```python
from build123d import *

# Parameters (mm, degrees)
F1_DEPTH = 63.5
F0_W     = 25.4
F0_H     = 19.05
F2_DEPTH = 25.4
F3_DEPTH = 7.9375
F4_R     = 6.35


with BuildPart() as f1:
    # F0 (on Top) → F1 (new body, symmetric)
    with BuildSketch(Plane.XY):
        Polygon((-41.275, -9.525), (41.275, -9.525), (41.275, 9.525), (22.225, 9.525), (-41.275, 9.525), align=None)
    extrude(amount=F1_DEPTH, both=True)

    # F0 (on Top) → F2 (join, symmetric)
    with BuildSketch(Plane.XY):
        with BuildLine():
            Line((22.225, 9.525), (41.275, 9.525))
            Line((41.275, 9.525), (41.275, 42.8379135305))
            ThreePointArc((41.275, 42.8379135305), (41.8183842247, 42.8658756442), (42.3624075254, 42.8752))
            Line((42.3624075254, 42.8752), (60.325, 42.8752))
            Line((60.325, 42.8752), (60.325, 61.9252))
            Line((60.325, 61.9252), (42.3624075254, 61.9252))
            add(Edge.make_bspline(
                [(41.3653767795, 61.9109655988), (41.6979264338, 61.916873269), (42.0302788073, 61.9216177836), (42.3624075254, 61.9252)],
                knots=[97.8694671613, 97.8694671613, 97.8694671613, 97.8694671613, 98.6964887806, 98.6964887806, 98.6964887806, 98.6964887806], degree=3))
            ThreePointArc((41.3653767795, 61.9109655988), (31.324788218, 60.1351752531), (22.225, 55.5350986883))
            Line((22.225, 55.5350986883), (22.225, 9.525))
        make_face()
        with Locations((73.025, 52.4002)):
            Rectangle(F0_W, F0_H)
    extrude(amount=F2_DEPTH, both=True)

    # F0 (on Top) → F3 (join, symmetric)
    with BuildSketch(Plane.XY):
        with BuildLine():
            add(Edge.make_bspline(
                [(-41.275, 9.525), (-40.1050332587, 44.223586325), (2.0115597622, 61.211853837), (41.3653767795, 61.9109655988)],
                knots=[0, 0, 0, 0, 97.8694671613, 97.8694671613, 97.8694671613, 97.8694671613], degree=3))
            Line((-41.275, 9.525), (22.225, 9.525))
            Line((22.225, 9.525), (22.225, 55.5350986883))
            ThreePointArc((22.225, 55.5350986883), (31.324788218, 60.1351752531), (41.3653767795, 61.9109655988))
        make_face()
    extrude(amount=F3_DEPTH, both=True)

    # F4
    f4_edges = [f1.edges().sort_by_distance(p)[0] for p in [
        (41.275, 0, 63.5),
        (-41.275, 0, 63.5),
        (-41.275, 0, -63.5),
        (41.275, 0, -63.5),
    ]]
    fillet(f4_edges, radius=F4_R)

    # F0 (on Top) → F5 (revolve)
    with BuildSketch(Plane.XY):
        Polygon((85.725, 61.9252), (85.725, 42.8752), (85.725, 38.1), (111.125, 38.1), (111.125, 66.675), (85.725, 66.675), align=None)
    revolve(axis=Axis((85.725, 52.3875, 0), (0, 1, 0)))


solid = f1.part
```
Verification items for the finished model (mm, model axes). A direction names the side the tool comes from. Coordinates: 2 decimals unless noted, no trailing zeros. Write each loop counter-clockwise with the first axis right and the second up, starting at its lowest first coordinate (ties: lowest second). Pieces come first, ordered by that corner, then holes. Notation, with made-up numbers: (2, -7.5) - (57, -7.5) arc R27 ccw to (57, 19.5) - close; hole circle Ø11 at (18, -15.5). An arc over 180 degrees is marked (long way). Write item = value, one per line.
Q1. Cross-section at C-C (x = 68.5). Enter the section's corners in (y, z) (3 decimals), plus the area to 3 significant figures.
Answer:
outline = (38.1, -18.667) - (42.875, -18.667) - (42.875, -25.4) - (61.925, -25.4) - (61.925, -18.667) - (66.675, -18.667) - (66.675, 18.667) - (61.925, 18.667) - (61.925, 25.4) - (42.875, 25.4) - (42.875, 18.667) - (38.1, 18.667) - close
area = 1,320 mm²
Q2. Material ranges on L1, parallel to Y at x = -23.5, z = -13 (3 decimals); L2, parallel to Z at x = 40, y = 42.5; L3, parallel to Z at x = -14, y = 18, recorded low to high. Write a range as from..to.
Answer:
L1 = -9.525..9.525
L2 = -25.4..25.4
L3 = -7.94..7.94
Q3. Cross-section at A-A (x = 52.5). Enter the section's corners in (y, z).
Answer:
outline = (42.88, -25.4) - (61.93, -25.4) - (61.93, 25.4) - (42.88, 25.4) - close
Q4. Go/stop test with flat-tipped pins: pin 1 Ø10 at (y, z) = (54, -13) entering from -X (3 decimals); pin 2 Ø21.5 at (x, z) = (61.5, 0) entering from -Y; pin 3 Ø8 at (y, z) = (14, -7.5) entering from +X (3 decimals). Record where each tip stops, or that it passes through.
Answer:
pin_1 = 22.225
pin_2 = 38.1
pin_3 = 41.275
Q5. Cross-section at B-B (z = -36). Enter the section's corners in (x, y) (3 decimals).
Answer:
outline = (-41.275, -9.525) - (41.275, -9.525) - (41.275, 9.525) - (-41.275, 9.525) - close
Q6. Access from +Z, -Z, +X, -X, +Y, -Y to the whole of each face (thin tool, end or side, straight path). Record for faces 1 (the face through (46, 48, -25.4)), 2 (the face through (22.225, 33, -17)), 3 (the face through (31.46, 60.18, 16.79)).
Answer:
face_1 = -Z, +X, -X, +Y
face_2 = -Z, -X, +Y
face_3 = +Z, -X, +Y
